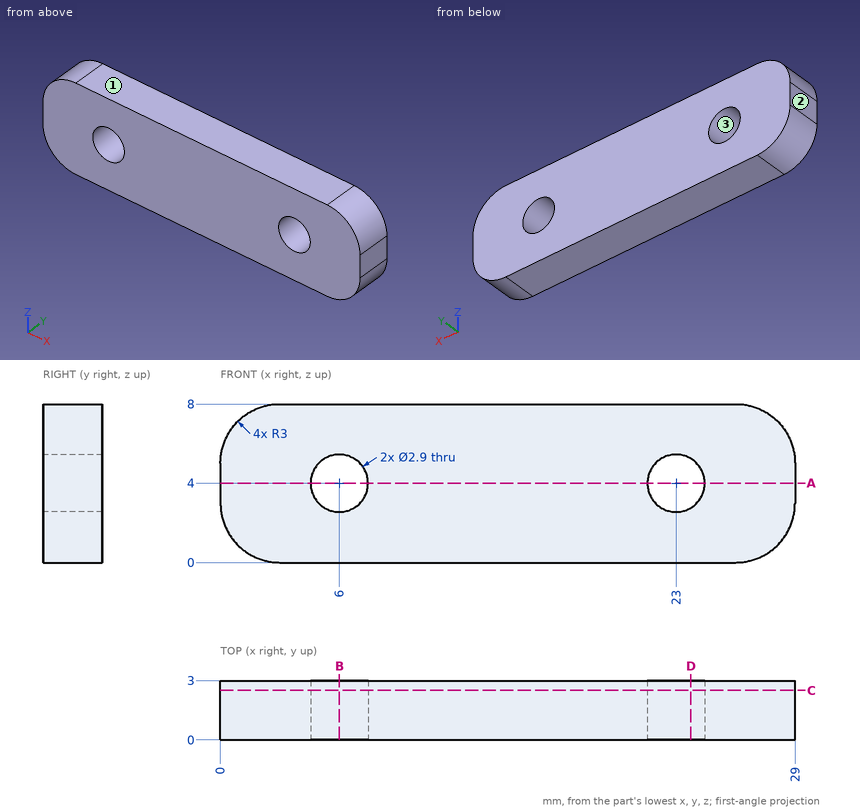
Verification items for this drawing (mm, ordinates from the low corner). Coordinates: 2 decimals unless noted, no trailing zeros. Order: outer loops, then holes, each group sorted by start corner. A loop starts at its lowest first (then second) coordinate and runs counter-clockwise, first axis right, second up. Notation, with made-up numbers: (-2, 24) - (33, 24) arc R33 cw to (33, 55) - close; hole circle Ø7 at (69, 0). An arc over 180 degrees is marked (long way). Answer in a Markdown table with one row per item. Add a question column.
1. Section check D-D (x = 23.75). Enter the section's corners in (y, z), plus the area to 3 significant figures.
2. Draft check along X on the marked faces 1, 2 and 3. Enter one of: +X half, -X half, draft (parallel to the pull), parting line (faces both ways), or undercut.
3. Gauge pin test, flat end, axial feed: pin 1 Ø4.5 at (x, z) = (6, 4) entering from +Y. Record the tip position at first contact, or that the pin passes through.
4. Section check B-B (x = 6). Enter the section's corners in (y, z), plus the area to 3 significant figures.
5. Section check A-A (z = 4). Enter the section's corners in (x, y), plus the area to 3 significant figures.
6. Material ranges on L1, parallel to X at y = 0.9, z = 4; L2, parallel to X at y = 2.2, z = 2.75; L3, parallel to Z at x = 23, y = 1.65, recorded low to high. Write a range as [from, to].
7. Section check C-C (y = 2.5). Enter the section's corners in (x, z), plus the area to 3 significant figures.
Data:
| question | item | result |
|---|---|---|
| 1 | outline | (0, 0) - (3, 0) - (3, 2.76) - (0, 2.76) - close; (0, 5.24) - (3, 5.24) - (3, 8) - (0, 8) - close |
| 1 | area | 16.6 mm² |
| 2 | face 1 | draft |
| 2 | face 2 | -X half |
| 2 | face 3 | undercut |
| 3 | pin 1 | stops at y = 3 |
| 4 | outline | (0, 0) - (3, 0) - (3, 2.55) - (0, 2.55) - close; (0, 5.45) - (3, 5.45) - (3, 8) - (0, 8) - close |
| 4 | area | 15.3 mm² |
| 5 | outline | (0, 0) - (4.55, 0) - (4.55, 3) - (0, 3) - close; (7.45, 0) - (21.55, 0) - (21.55, 3) - (7.45, 3) - close; (24.45, 0) - (29, 0) - (29, 3) - (24.45, 3) - close |
| 5 | area | 69.6 mm² |
| 6 | L1 | x = [0, 4.55], [7.45, 21.55], [24.45, 29] |
| 6 | L2 | x = [0.01, 5.27], [6.73, 22.27], [23.73, 28.99] |
| 6 | L3 | z = [0, 2.55], [5.45, 8] |
| 7 | outline | (0, 3) arc R3 ccw to (3, 0) - (26, 0) arc R3 ccw to (29, 3) - (29, 5) arc R3 ccw to (26, 8) - (3, 8) arc R3 ccw to (0, 5) - close; hole circle Ø2.9 at (6, 4); hole circle Ø2.9 at (23, 4) |
| 7 | area | 211 mm² |
